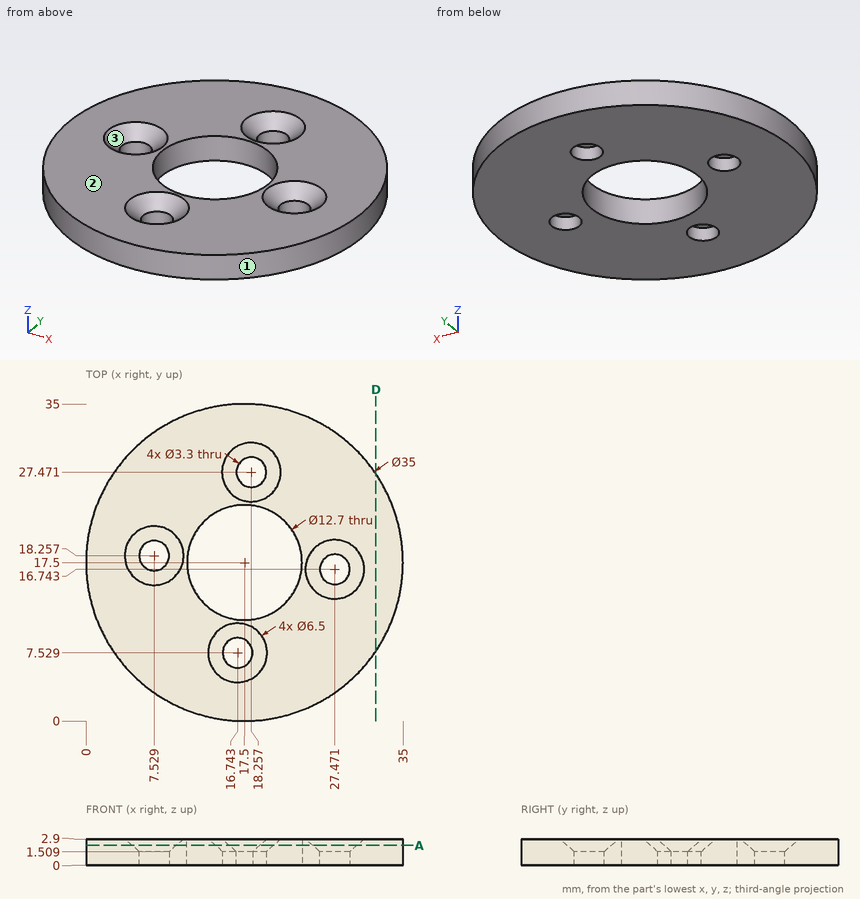
Input: dimensioned drawing with shaded views. Units: mm. Origin: part minimum x, y, z. Give positions to 0.01 mm unless a question says otherwise; leave off trailing zeros. Write each loop counter-clockwise with the first axis right and the second up, starting at its lowest first coordinate (ties: lowest second). Pieces come first, ordered by that corner, then holes. Notation, with made-up numbers: M -36,62 L -9,62 A8 ccw -9,73 Z; hole C 43,84.25 d5. An arc over 180 degrees is marked long. Return JSON: item names as keys, results as strings. Group by question number.
1) Cut plane A-A, the plane z = 2.2. Give the number of separate pieces and of enclosed holes in the cut face.
2) Cut plane D-D, the plane x = 32. Output: boundary loops of the cut face in (y, z).
3) Material intervals for line 1 along Y through (x, z) = (18.5, 0.5); line 2 along X through (y, z) = (8, 1.25) (1 decimal); line 3 along Y through (x, z) = (21, 1.6) (1 decimal), sorted ascending. Write a range as [from, to].
4) Pin query (flat end, axial travel): P1, Ø2, axis at x = 18.26, y = 27.47, coming from the -Z side; P2, Ø1, axis at x = 11, z = 0.5, coming from the +Y side; P3, Ø1.5, axis at y = 19.5, z = 1, coming from the -X side (1 decimal); P4, Ø5.5, axis at x = 27.47, y = 16.74, coming from the +Z side. Return the tip coordinate at first contact, or that it passes through.
5) Pull-direction query (Y, two-part tool) for the marked faces 1, 2 and 3; classes: pulls with the +Y half, pulls with the -Y half, needs draft (parallel to the pull), parting line crosses it, or undercut.
Recorded:
{
 "1": {"separate pieces": "1", "enclosed holes": "5"},
 "2": {"outline": "M 7.7,0 L 27.3,0 L 27.3,2.9 L 7.7,2.9 Z"},
 "3": {"line 1": "y = [0.03, 11.23], [23.77, 25.84], [29.1, 34.97]", "line 2": "x = [2.8, 15.2], [18.3, 32.2]", "line 3": "y = [0.4, 12.2], [22.8, 34.6]"},
 "4": {"P1": "passes through", "P2": "stops at y = 33.94", "P3": "stops at x = 0", "P4": "stops at z = 2.47"},
 "5": {"face 1": "parting line crosses it", "face 2": "needs draft", "face 3": "undercut"}
}
